Here's how the part is built. I have some questions about the finished solid (model axes, mm). A direction names the side the tool comes from. Round coordinates to 2 decimals unless told otherwise and drop trailing zeros. Write each loop counter-clockwise with the first axis right and the second up, starting at its lowest first coordinate (ties: lowest second). Pieces come first, ordered by that corner, then holes. Notation, with made-up numbers: (14, -38) - (35, -38) arc R14 cw to (35, -22) - close; hole circle Ø7 at (38.5, 87.5). An arc over 180 degrees is marked (long way). One line per question, with ' | ' between items. Start each with the question number.
(1) For faces 1 (the flat face through (0, 4, 13)), 2 (the cylindrical face through (4.84, 14.306, 1.265)), 3 (the cylindrical face through (-1.265, 14.306, -4.838)), which set-ups out of +Z, -Z, +X, -X, +Y, -Y let a thin tool reach every point of the face, with its end or its side?
(2) Imagine slicing it at C-C (x = 0). Write out the boundary of the cut face in (y, z).
(3) Imagine slicing it at B-B (y = 2.5). Write out the boundary of the cut face in (x, z).
(4) Thinking about a two-plate mould opening in X: for faces 4 (the cylindrical face through (20.73, 1.97, -0.33)), 5 (the flat face through (13.39, 1.97, 8.49)), 6 (the cylindrical face through (0.1, 2, 13.5)), which applies, pulls with the +X half, pulls with the -X half, needs draft (parallel to the pull), parting line crosses it, or undercut?
(5) Will these pins go through, and if not, where does the flat tip stop? pin 1 (10 mm diameter, centred on x = 11, z = 6.5, fed in from +Y); pin 2 (1.5 mm diameter, centred on x = -7, y = 4.5, fed in from +Z); pin 3 (4 mm diameter, centred on x = 0, y = 13.5, fed in from -Z); pin 4 (4 mm diameter, centred on x = 18.25, z = 0, fed in from -Y).
(6) Imagine slicing it at D-D (y = 13.5). Write out the boundary of the cut face in (x, z).
(7) If I drill on L1, parallel to X at y = 2.8, z = 0; L2, parallel to X at y = 5.75, z = 0; L3, parallel to X at y = 1, z = 1, over which ranges is the centre line in solid material (lowest first)?
(8) Imagine slicing it at A-A (z = 0). Write out the boundary of the cut face in (x, y).
from build123d import *

# Parameters (mm, degrees)
SKETCH1_R           = 2.5
SKETCH1_R_2         = 4
BOSS_EXTRUDE1_DEPTH = 4
SKETCH2_R           = 12.5
SKETCH2_R_2         = 4
BOSS_EXTRUDE2_DEPTH = 6
SKETCH3_R           = 6
SKETCH3_R_2         = 4
BOSS_EXTRUDE3_DEPTH = 7
SKETCH4_R           = 1.5
CUT_EXTRUDE1_DEPTH  = 33.176272314


with BuildPart() as part:
    # Sketch1 → Boss-Extrude1 (new body)
    with BuildSketch(Plane(origin=(0, 0, 0), x_dir=(1, 0, 0), z_dir=(0, 1, 0))):
        with BuildLine():
            Line((-20.660958904, 4.943407445), (-5.917808219, 12.133818273))
            ThreePointArc((-5.917808219, 12.133818273), (0, 13.5), (5.917808219, 12.133818273))
            Line((5.917808219, 12.133818273), (20.660958904, 4.943407445))
            ThreePointArc((20.660958904, 4.943407445), (23.75, 0), (20.660958904, -4.943407445))
            Line((20.660958904, -4.943407445), (5.917808219, -12.133818273))
            ThreePointArc((5.917808219, -12.133818273), (0, -13.5), (-5.917808219, -12.133818273))
            Line((-5.917808219, -12.133818273), (-20.660958904, -4.943407445))
            ThreePointArc((-20.660958904, -4.943407445), (-23.75, 0), (-20.660958904, 4.943407445))
        make_face()
        with Locations(Location((18.25, 0, 0), (0, 0, 270))):
            Circle(SKETCH1_R, mode=Mode.SUBTRACT)
        with Locations(Location((-18.25, 0, 0), (0, 0, 90))):
            Circle(SKETCH1_R, mode=Mode.SUBTRACT)
        with Locations(Location((0, 0, 0), (0, 0, 270))):
            Circle(SKETCH1_R_2, mode=Mode.SUBTRACT)
    extrude(amount=BOSS_EXTRUDE1_DEPTH)

    # Sketch2 → Boss-Extrude2 (add)
    with BuildSketch(Plane(origin=(0, 4, 0), x_dir=(1, 0, 0), z_dir=(0, 1, 0))):
        with Locations(Location((0, 0, 0), (0, 0, 270))):
            Circle(SKETCH2_R)
        with Locations(Location((0, 0, 0), (0, 0, 270))):
            Circle(SKETCH2_R_2, mode=Mode.SUBTRACT)
    extrude(amount=BOSS_EXTRUDE2_DEPTH)

    # Sketch3 → Boss-Extrude3 (add)
    with BuildSketch(Plane(origin=(0, 10, 0), x_dir=(1, 0, 0), z_dir=(0, 1, 0))):
        with Locations(Location((0, 0, 0), (0, 0, 270))):
            Circle(SKETCH3_R)
        with Locations(Location((0, 0, 0), (0, 0, 270))):
            Circle(SKETCH3_R_2, mode=Mode.SUBTRACT)
    extrude(amount=BOSS_EXTRUDE3_DEPTH)

    # Sketch4 → Cut-Extrude1 (cut, through all)
    with BuildSketch(Plane.XY):
        with Locations(Location((0, 13.5, 0), (0, 0, 90))):
            Circle(SKETCH4_R)
    cut_extrude1 = extrude(amount=-CUT_EXTRUDE1_DEPTH, mode=Mode.SUBTRACT)

    # Mirror1: Cut-Extrude1 across plane
    add(cut_extrude1.mirror(Plane(origin=(0, 0, 0), x_dir=(-0.7071067811865478, 0, 0.7071067811865472), z_dir=(0.7071067811865475, 0, 0.7071067811865477))), mode=Mode.SUBTRACT)


solid = part.part
Check sheet entries:
1) face 1: +Y | face 2: +X | face 3: -Z
2) outline: (0, -13.5) - (4, -13.5) - (4, -12.5) - (10, -12.5) - (10, -6) - (12, -6) - (12, -4) - (0, -4) - close; (0, 4) - (17, 4) - (17, 6) - (10, 6) - (10, 12.5) - (4, 12.5) - (4, 13.5) - (0, 13.5) - close; (15, -6) - (17, -6) - (17, -4) - (15, -4) - close
3) outline: (-20.66, -4.94) - (-5.92, -12.13) arc R13.5 ccw to (5.92, -12.13) - (20.66, -4.94) arc R5.5 ccw to (20.66, 4.94) - (5.92, 12.13) arc R13.5 ccw to (-5.92, 12.13) - (-20.66, 4.94) arc R5.5 ccw to start; hole circle Ø5 at (-18.25, 0); hole circle Ø8 at (0, 0); hole circle Ø5 at (18.25, 0)
4) face 4: undercut | face 5: pulls with the +X half | face 6: parting line crosses it
5) pin 1: y = 10 | pin 2: z = 11.88 | pin 3: z = -6 | pin 4: through
6) outline: (-1.5, -5.81) - (-1.5, -3.71) arc R4 cw (long way) to (3.71, 1.5) - (5.81, 1.5) arc R6 ccw (long way) to start; (1.5, -5.81) arc R6 ccw to (5.81, -1.5) - (3.71, -1.5) arc R4 cw to (1.5, -3.71) - close
7) L1: -23.75 to -20.75, -15.75 to -4, 4 to 15.75, 20.75 to 23.75 | L2: -12.5 to -4, 4 to 12.5 | L3: -23.66 to -20.54, -15.96 to -3.87, 3.87 to 15.96, 20.54 to 23.66
8) outline: (-23.75, 0) - (-20.75, 0) - (-20.75, 4) - (-23.75, 4) - close; (-15.75, 0) - (-4, 0) - (-4, 17) - (-6, 17) - (-6, 10) - (-12.5, 10) - (-12.5, 4) - (-15.75, 4) - close; (4, 0) - (15.75, 0) - (15.75, 4) - (12.5, 4) - (12.5, 10) - (6, 10) - (6, 12) - (4, 12) - close; (4, 15) - (6, 15) - (6, 17) - (4, 17) - close; (20.75, 0) - (23.75, 0) - (23.75, 4) - (20.75, 4) - close
